from build123d import *

# Parameters (mm, degrees)
F1_DEPTH = 3


with BuildPart() as f1:
    # F0 (on Top) → F1 (new body)
    with BuildSketch(Plane.XY):
        Polygon((57.5, 57.5), (55.732233047, 57.5), (1.25, 3.017766953), (1.25, 1.25), align=None)
        Polygon((-55.732233047, -57.5), (-58.232233047, -60), (58.232233047, -60), (55.732233047, -57.5), (1.25, -57.5), (-1.25, -57.5), align=None)
        Polygon((57.5, -1.25), (57.5, 1.25), (3.017766953, 1.25), (1.767766953, 0), (3.017766953, -1.25), align=None)
        Polygon((1.25, 57.5), (-1.25, 57.5), (-1.25, 3.017766953), (0, 1.767766953), (1.25, 3.017766953), align=None)
        Polygon((-1.25, 1.25), (-57.5, 57.5), (-57.5, 55.732233047), (-3.017766953, 1.25), align=None)
        Polygon((-57.5, 55.732233047), (-60, 58.232233047), (-60, -58.232233047), (-57.5, -55.732233047), (-57.5, -1.25), (-57.5, 1.25), align=None)
        Polygon((-1.25, -1.25), (-57.5, -57.5), (-55.732233047, -57.5), (-1.25, -3.017766953), align=None)
        Polygon((-1.25, -3.017766953), (-1.25, -57.5), (1.25, -57.5), (1.25, -3.017766953), (0, -1.767766953), align=None)
        Polygon((-3.017766953, -1.25), (-57.5, -55.732233047), (-57.5, -57.5), (-1.25, -1.25), align=None)
        Polygon((58.232233047, 60), (-58.232233047, 60), (-55.732233047, 57.5), (-1.25, 57.5), (1.25, 57.5), (55.732233047, 57.5), align=None)
        Polygon((-3.017766953, 1.25), (-57.5, 1.25), (-57.5, -1.25), (-3.017766953, -1.25), (-1.767766953, 0), align=None)
        Polygon((57.5, 55.732233047), (57.5, 57.5), (1.25, 1.25), (3.017766953, 1.25), align=None)
        Polygon((60, -58.232233047), (60, 58.232233047), (57.5, 55.732233047), (57.5, 1.25), (57.5, -1.25), (57.5, -55.732233047), align=None)
        Polygon((3.017766953, 1.25), (1.25, 1.25), (1.25, 0.517766953), (1.767766953, 0), align=None)
        Polygon((57.5, -57.5), (57.5, -55.732233047), (3.017766953, -1.25), (1.25, -1.25), align=None)
        Polygon((-1.25, 3.017766953), (-1.25, 1.25), (-0.517766953, 1.25), (0, 1.767766953), align=None)
        Polygon((-0.517766953, -1.25), (-1.25, -1.25), (-1.25, -3.017766953), (0, -1.767766953), align=None)
        Polygon((-58.232233047, 60), (-60, 60), (-57.5, 57.5), (-55.732233047, 57.5), align=None)
        Polygon((60, 60), (58.232233047, 60), (55.732233047, 57.5), (57.5, 57.5), align=None)
        Polygon((-57.5, -57.5), (-60, -60), (-58.232233047, -60), (-55.732233047, -57.5), align=None)
        Polygon((55.732233047, -57.5), (58.232233047, -60), (60, -60), (57.5, -57.5), align=None)
        Polygon((-57.5, 57.5), (-60, 60), (-60, 58.232233047), (-57.5, 55.732233047), align=None)
        Polygon((-57.5, -55.732233047), (-60, -58.232233047), (-60, -60), (-57.5, -57.5), align=None)
        Polygon((60, -60), (60, -58.232233047), (57.5, -55.732233047), (57.5, -57.5), align=None)
        Polygon((1.25, -3.017766953), (1.25, -1.25), (0.517766953, -1.25), (0, -1.767766953), align=None)
        Polygon((1.25, -0.517766953), (1.25, -1.25), (3.017766953, -1.25), (1.767766953, 0), align=None)
        Polygon((1.25, 1.25), (1.25, 3.017766953), (0, 1.767766953), (0.517766953, 1.25), align=None)
        Polygon((-55.732233047, 57.5), (-57.5, 57.5), (-1.25, 1.25), (-1.25, 3.017766953), align=None)
        Polygon((-1.25, 0.517766953), (-1.25, 1.25), (-3.017766953, 1.25), (-1.767766953, 0), align=None)
        Polygon((1.25, -3.017766953), (55.732233047, -57.5), (57.5, -57.5), (1.25, -1.25), align=None)
        Polygon((-1.767766953, 0), (-3.017766953, -1.25), (-1.25, -1.25), (-1.25, -0.517766953), align=None)
        Polygon((0, 0), (-0.8838834765, 0.8838834765), (-1.25, 0.517766953), (-1.25, -0.517766953), (-0.8838834765, -0.8838834765), align=None)
        Polygon((-0.517766953, 1.25), (-0.8838834765, 0.8838834765), (0, 0), (0.8838834765, 0.8838834765), (0.517766953, 1.25), align=None)
        Polygon((-0.8838834765, -0.8838834765), (-1.25, -1.25), (-0.517766953, -1.25), align=None)
        Polygon((-1.25, -0.517766953), (-1.25, 0.517766953), (-1.767766953, 0), align=None)
        Polygon((-0.517766953, 1.25), (-1.25, 1.25), (-0.8838834765, 0.8838834765), align=None)
        Polygon((1.25, -0.517766953), (0.8838834765, -0.8838834765), (1.25, -1.25), align=None)
        Polygon((1.25, 1.25), (0.517766953, 1.25), (0.8838834765, 0.8838834765), align=None)
        Polygon((60, 58.232233047), (60, 60), (57.5, 57.5), (57.5, 55.732233047), align=None)
        Polygon((0.517766953, -1.25), (-0.517766953, -1.25), (0, -1.767766953), align=None)
        Polygon((0.8838834765, -0.8838834765), (0, 0), (-0.8838834765, -0.8838834765), (-0.517766953, -1.25), (0.517766953, -1.25), align=None)
        Polygon((0.8838834765, 0.8838834765), (0, 0), (0.8838834765, -0.8838834765), (1.25, -0.517766953), (1.25, 0.517766953), align=None)
        Polygon((0, 1.767766953), (-0.517766953, 1.25), (0.517766953, 1.25), align=None)
        Polygon((1.767766953, 0), (1.25, 0.517766953), (1.25, -0.517766953), align=None)
        Polygon((1.25, -1.25), (0.8838834765, -0.8838834765), (0.517766953, -1.25), align=None)
        Polygon((-0.8838834765, 0.8838834765), (-1.25, 1.25), (-1.25, 0.517766953), align=None)
        Polygon((1.25, 0.517766953), (1.25, 1.25), (0.8838834765, 0.8838834765), align=None)
        Polygon((-0.8838834765, -0.8838834765), (-1.25, -0.517766953), (-1.25, -1.25), align=None)
    extrude(amount=F1_DEPTH)


solid = f1.part
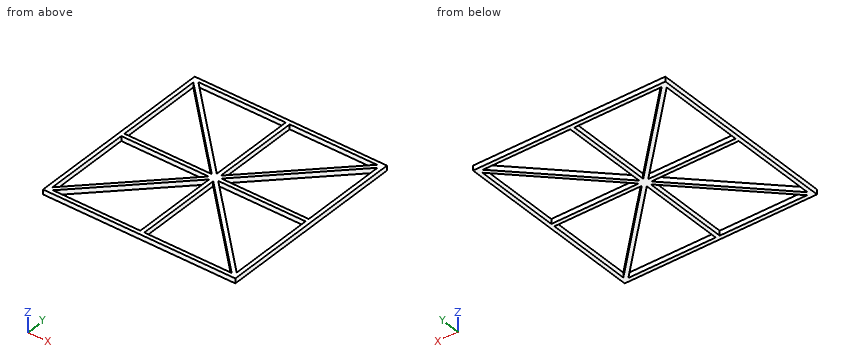
Build history of the part. All positions in model axes, mm. Give positions to 0.01 mm unless a question says otherwise; leave off trailing zeros. Order: outer loops, then holes, each group sorted by start corner. A loop starts at its lowest first (then second) coordinate and runs counter-clockwise, first axis right, second up. Notation, with made-up numbers: M 66.25,51 L 119.25,51 A36 ccw 119.25,85 Z; hole C -25,-10 d4. An arc over 180 degrees is marked long. Put each result on its own line as item: value.
Item 1: Slice it at A-A, the plane z = 2.2. Give the number of separate pieces and of enclosed holes in the cut face, plus the area to 3 significant figures.
From the geometry:
separate pieces: 1
enclosed holes: 8
area: 2,530 mm2
Item 2: Probe line 1 (Y direction, x = 36, z = 1.95); line 2 (Y direction, x = 28.5, z = 0.9); line 3 (X direction, y = 29.5, z = 2.4). List the from-to ranges inside material, lowest first. Write a range as [from, to].
From the geometry:
line 1: y = [-60, -57.5], [-37.77, -34.23], [-1.25, 1.25], [34.23, 37.77], [57.5, 60]
line 2: y = [-60, -57.5], [-30.27, -26.73], [-1.25, 1.25], [26.73, 30.27], [57.5, 60]
line 3: x = [-60, -57.5], [-31.27, -27.73], [-1.25, 1.25], [27.73, 31.27], [57.5, 60]
Item 3: Slice it at B-B, the plane y = 12. Write the cut outline in (x, z).
From the geometry:
outline: M -60,0 L -57.5,0 L -57.5,3 L -60,3 Z; M -13.77,0 L -10.23,0 L -10.23,3 L -13.77,3 Z; M -1.25,0 L 1.25,0 L 1.25,3 L -1.25,3 Z; M 10.23,0 L 13.77,0 L 13.77,3 L 10.23,3 Z; M 57.5,0 L 60,0 L 60,3 L 57.5,3 Z
Item 4: Slice it at C-C, the plane x = 32.5. Write the cut outline in (y, z), plus the area to 3 significant figures.
From the geometry:
outline: M -60,0 L -57.5,0 L -57.5,3 L -60,3 Z; M -34.27,0 L -30.73,0 L -30.73,3 L -34.27,3 Z; M -1.25,0 L 1.25,0 L 1.25,3 L -1.25,3 Z; M 30.73,0 L 34.27,0 L 34.27,3 L 30.73,3 Z; M 57.5,0 L 60,0 L 60,3 L 57.5,3 Z
area: 43.7 mm2
Item 5: Flat gauge pin, fed straight in: pin 1 Ø6 at (x, y) = (14, -16.5) entering from -Z. Where does the tip first touch, or does it go through?
From the geometry:
pin 1: stops at z = 0
